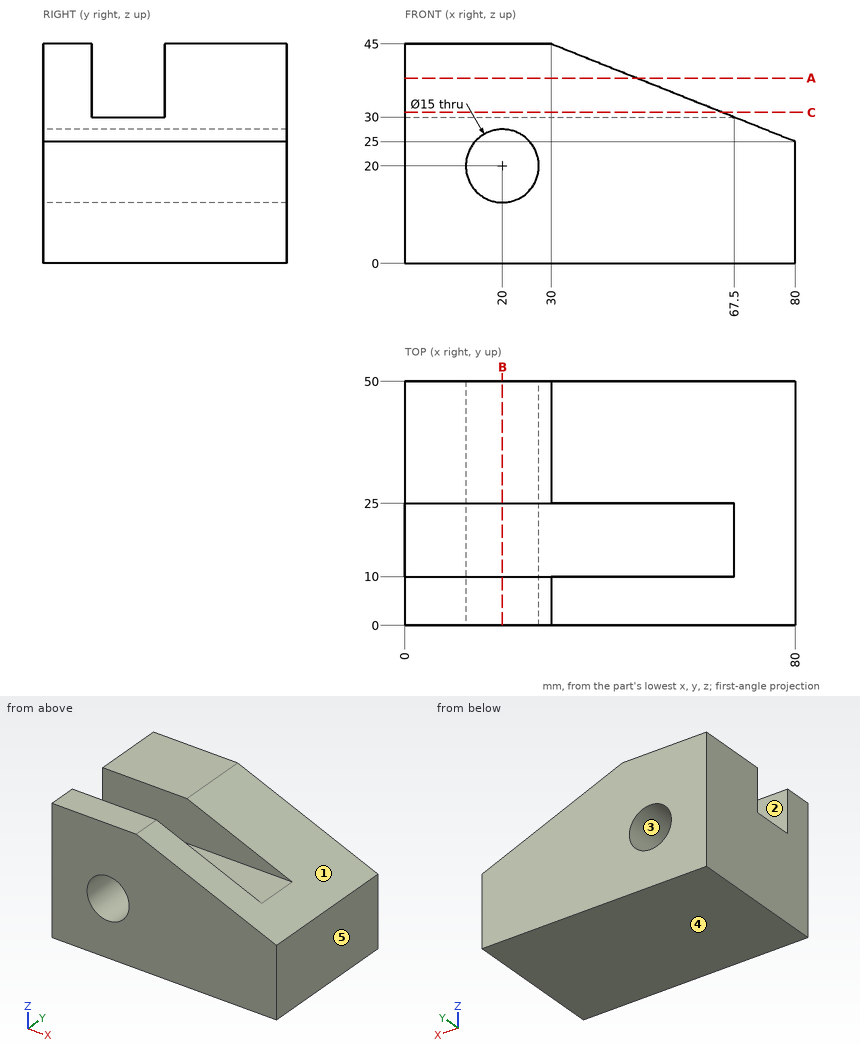
Verification items for this drawing (mm, ordinates from the low corner). A direction names the side the tool comes from. Coordinates: 2 decimals unless noted, no trailing zeros. Loops run counter-clockwise (first coordinate to the right, second up) from the corner with the lowest first, then second, coordinate; pieces in that order, holes last.
Item 1: Go/stop test with flat-tipped pins: pin 1 Ø6 at (x, y) = (54.5, 38.5) entering from +Z; pin 2 Ø1.5 at (x, y) = (68.5, 10) entering from +Z; pin 3 Ø8 at (x, z) = (63.5, 38) entering from -Y. Record where each tip stops, or that it passes through.
Item 2: Access from +Z, -Z, +X, -X, +Y, -Y to the whole of each face (thin tool, end or side, straight path). Record for the marked faces 1 and 2.
Item 3: Sectioned sample at A-A, the plane z = 38. Record the boundary of the cut face in (x, y).
Item 4: Sectioned sample at C-C, the plane z = 31. Record the boundary of the cut face in (x, y).
Item 5: Release check for a two-part mould opening along Z. For the marked faces 3, 4 and 5 record: released by +Z, released by -Z, zero draft, split by the parting line, or undercut.
Item 6: Sectioned sample at B-B, the plane x = 20. Record the boundary of the cut face in (y, z).
Item 7: Thickness scan on line 1 (Z direction, x = 20, y = 23); line 2 (Z direction, x = 20, y = 25.5); line 3 (Y direction, x = 9, z = 40.5). Record the ranges inside material, lowest first.
Check result:
1. pin 1: stops at z = 36.4
1. pin 2: stops at z = 29.9
1. pin 3: passes through
2. face 1: +Z, +X, +Y, -Y
2. face 2: +Z, +X, -X
3. outline: (0, 0) - (47.5, 0) - (47.5, 10) - (0, 10) - close; (0, 25) - (47.5, 25) - (47.5, 50) - (0, 50) - close
4. outline: (0, 0) - (65, 0) - (65, 10) - (0, 10) - close; (0, 25) - (65, 25) - (65, 50) - (0, 50) - close
5. face 3: undercut
5. face 4: released by -Z
5. face 5: zero draft
6. outline: (0, 0) - (50, 0) - (50, 12.5) - (0, 12.5) - close; (0, 27.5) - (50, 27.5) - (50, 45) - (25, 45) - (25, 30) - (10, 30) - (10, 45) - (0, 45) - close
7. line 1: z = 0 to 12.5, 27.5 to 30
7. line 2: z = 0 to 12.5, 27.5 to 45
7. line 3: y = 0 to 10, 25 to 50
